The model under review builds one solid part; all positions refer to its coordinate system, in mm. Face numbers are marked on the shaded views. A direction names the side the tool comes from. Coordinates: 2 decimals unless noted, no trailing zeros. Order: outer loops, then holes, each group sorted by start corner. A loop starts at its lowest first (then second) coordinate and runs counter-clockwise, first axis right, second up. Notation, with made-up numbers: (49.5, 66) -> (71.5, 66) arc R25 cw to (71.5, 80) -> close; hole circle Ø4 at (82, -24.75). An arc over 180 degrees is marked (long way). Use one line per item in the form item = value.
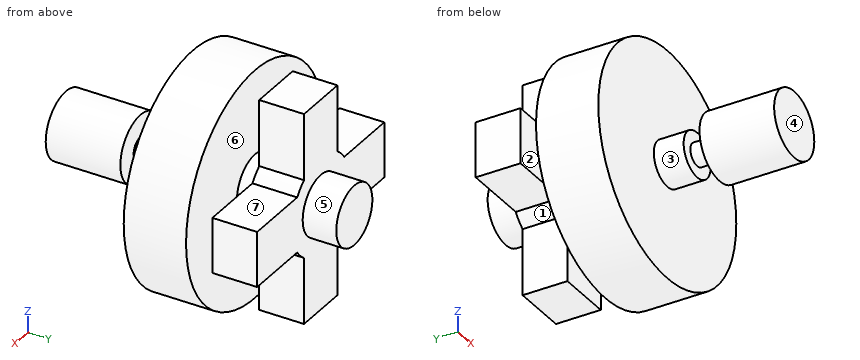
Autodesk Inventor part; units mm, degrees
ref_plane "YZ Plane" through (0, 0, 0) normal (1, 0, 0) x (0, 1, 0)
ref_plane "XZ Plane" through (0, 0, 0) normal (0, 1, 0) x (-1, 0, 0)
ref_plane "XY Plane" through (0, 0, 0) normal (0, 0, 1) x (1, 0, 0)
sketch "Sketch1" plane through (0, 0, 0) normal (0, 1, 0) x (-1, 0, 0)
  circle A0 centre (0, 0) radius 15.3
  dimension "d0" = 30.6
extrude "Extrusion1" add sketch "Sketch1" against normal blind 8.35
sketch "Sketch2" plane through (0, 0, 0) normal (0, 1, 0) x (1, 0, 0)
  circle A0 centre (0, 0) radius 4
  dimension "d3" = 8
extrude "Extrusion2" add sketch "Sketch2" along normal blind 2.8
sketch "Sketch3" plane through (0, 2.8, 0) normal (0, 1, 0) x (1, 0, 0)
  line L0 (-3.7, 14.1) -> (3.7, 14.1)
  line L1 (3.7, -14.1) -> (-3.7, -14.1)
  line L2 (-3.7, 14.1) -> (3.7, -14.1) construction
  line L3 (3.7, 14.1) -> (-3.7, -14.1) construction
  line L4 (14.1, 3.7) -> (14.1, -3.7)
  line L5 (-14.1, -3.7) -> (-14.1, 3.7)
  line L6 (-14.1, 3.7) -> (14.1, -3.7) construction
  line L7 (14.1, 3.7) -> (-14.1, -3.7) construction
  line L8 (3.7, 14.1) -> (3.7, 5.2221)
  line L9 (3.7, -5.2221) -> (3.7, -14.1)
  line L10 (14.1, -3.7) -> (5.2221, -3.7)
  line L11 (-5.2221, -3.7) -> (-14.1, -3.7)
  line L12 (-14.1, 3.7) -> (-5.2221, 3.7)
  line L13 (5.2221, 3.7) -> (14.1, 3.7)
  line L14 (-3.7, -14.1) -> (-3.7, -5.2221)
  line L15 (-3.7, 5.2221) -> (-3.7, 14.1)
  arc A0 (3.7, -5.2221) -> (5.2221, -3.7) centre (0, 0) ccw
  arc A1 (-5.2221, -3.7) -> (-3.7, -5.2221) centre (0, 0) ccw
  arc A2 (5.2221, 3.7) -> (3.7, 5.2221) centre (0, 0) ccw
  arc A3 (-3.7, 5.2221) -> (-5.2221, 3.7) centre (0, 0) ccw
  dimension "d6" = 7.4
  dimension "d7" = 28.2
  dimension "d8" = 28.2
  dimension "d9" = 7.4
extrude "Extrusion3" add sketch "Sketch3" along normal blind 6
sketch "Sketch4" plane through (0, 8.8, 0) normal (0, 1, 0) x (1, 0, 0)
  circle A0 centre (0, 0) radius 4
  dimension "d13" = 8
extrude "Extrusion4" add sketch "Sketch4" along normal blind 4.5
sketch "Sketch5" plane through (0, -8.35, 0) normal (0, -1, 0) x (1, 0, 0)
  circle A0 centre (0, 0) radius 4
  circle A1 centre (0, 0) radius 3
  dimension "d16" = 6
extrude "Extrusion5" add sketch "Sketch5" along normal blind 4 contours A1
sketch "Sketch6" plane through (0, -12.35, 0) normal (0, -1, 0) x (1, 0, 0)
  circle A0 centre (0, 0) radius 1.5
  dimension "d19" = 3
extrude "Extrusion6" add sketch "Sketch6" along normal blind 13
sketch "Sketch7" plane through (0, -25.35, 0) normal (0, -1, 0) x (1, 0, 0)
  circle A0 centre (0, 0) radius 4.45
  dimension "d22" = 8.9
extrude "Extrusion7" add sketch "Sketch7" against normal blind 10
properties part number "BrImp_Motormodel" material "Aluminum 6061"
Item 1: To check wall thickness, follow L1, parallel to Y at x = 2, z = -9.5; L2, parallel to Y at x = 9, z = 8.5; L3, parallel to Z at x = -0.5, y = -5.5. State the ranges of each line that lie inside material, in increasing order. Write a range as from..to.
Results found:
L1 = -8.35..0, 2.8..8.8
L2 = -8.35..0
L3 = -15.29..15.29
Item 2: Draft analysis for pull direction Y (two halves, no side actions). For the marked faces 1, 2, 3 and 4, state which applies: released by +Y, released by -Y, zero draft, split by the parting line, or undercut.
Results found:
face_1 = zero draft
face_2 = undercut
face_3 = undercut
face_4 = released by -Y
Item 3: Clearance check with flat-ended pins moving along their axes: pin 1 (3 mm diameter, centred on y = 6, z = -10, fed in from -X); pin 2 (3 mm diameter, centred on x = -7.5, y = 5.5, fed in from +Z); pin 3 (1.8 mm diameter, centred on y = 5, z = 8, fed in from +X). State where each tip first meets the part, or that it passes through.
Results found:
pin_1 = -3.7
pin_2 = 3.7
pin_3 = 3.7
Item 4: We need section B-B (x = 6). Write out the cut boundary in (y, z).
Results found:
outline = (-8.35, -14.07) -> (0, -14.07) -> (0, 14.07) -> (-8.35, 14.07) -> close; (2.8, -3.7) -> (8.8, -3.7) -> (8.8, 3.7) -> (2.8, 3.7) -> close
Item 5: We need section A-A (x = 0). Write out the cut boundary in (y, z), plus the area to 3 significant figures.
Results found:
outline = (-25.35, -4.45) -> (-15.35, -4.45) -> (-15.35, -1.5) -> (-12.35, -1.5) -> (-12.35, -3) -> (-8.35, -3) -> (-8.35, -15.3) -> (0, -15.3) -> (0, -4) -> (2.8, -4) -> (2.8, -14.1) -> (8.8, -14.1) -> (8.8, -4) -> (13.3, -4) -> (13.3, 4) -> (8.8, 4) -> (8.8, 14.1) -> (2.8, 14.1) -> (2.8, 4) -> (0, 4) -> (0, 15.3) -> (-8.35, 15.3) -> (-8.35, 3) -> (-12.35, 3) -> (-12.35, 1.5) -> (-15.35, 1.5) -> (-15.35, 4.45) -> (-25.35, 4.45) -> close
area = 605 mm²
Item 6: We need section C-C (z = 12). Write out the cut boundary in (x, y), plus the area to 3 significant figures.
Results found:
outline = (-9.49, -8.35) -> (9.49, -8.35) -> (9.49, 0) -> (-9.49, 0) -> close; (-3.7, 2.8) -> (3.7, 2.8) -> (3.7, 8.8) -> (-3.7, 8.8) -> close
area = 203 mm²
Item 7: We need section D-D (z = 0). Write out the cut boundary in (x, y), plus the area to 3 significant figures.
Results found:
outline = (-15.3, -8.35) -> (-3, -8.35) -> (-3, -12.35) -> (-1.5, -12.35) -> (-1.5, -15.35) -> (-4.45, -15.35) -> (-4.45, -25.35) -> (4.45, -25.35) -> (4.45, -15.35) -> (1.5, -15.35) -> (1.5, -12.35) -> (3, -12.35) -> (3, -8.35) -> (15.3, -8.35) -> (15.3, 0) -> (4, 0) -> (4, 2.8) -> (14.1, 2.8) -> (14.1, 8.8) -> (4, 8.8) -> (4, 13.3) -> (-4, 13.3) -> (-4, 8.8) -> (-14.1, 8.8) -> (-14.1, 2.8) -> (-4, 2.8) -> (-4, 0) -> (-15.3, 0) -> close
area = 605 mm²
Item 8: Tool access review of the marked faces 5, 6 and 7: name each direction out of +Z, -Z, +X, -X, +Y, -Y from which nothing blocks a thin tool from reaching the whole face with its end or side.
Results found:
face_5 = +Y
face_6 = none
face_7 = +Z, +X, +Y
